For this review, use the dimensioned drawing (mm, ordinates from the lowest corner) and the shaded views. Coordinates: 2 decimals unless noted, no trailing zeros. Loops run counter-clockwise (first coordinate to the right, second up) from the corner with the lowest first, then second, coordinate; pieces in that order, holes last. Notation, with made-up numbers: M 11.25,22 L 35.25,22 A7 ccw 35.25,32 Z; hole C 72,-2.5 d10. An arc over 180 degrees is marked long. One line per item, written item: value.
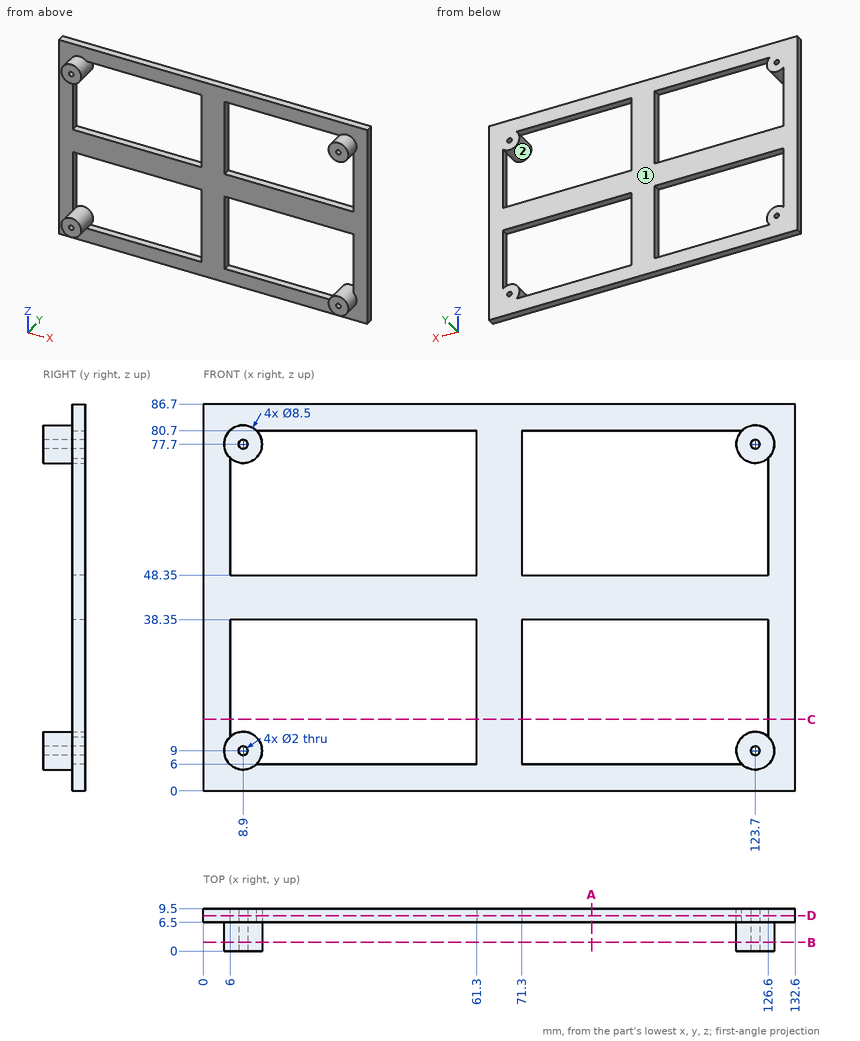
(1) Add section B-B on y = 2. State the section outline as (x, z) points.
Checks:
outline: C 8.9,9 d8.5; C 8.9,77.7 d8.5; C 123.7,9 d8.5; C 123.7,77.7 d8.5; hole C 8.9,9 d2; hole C 8.9,77.7 d2; hole C 123.7,9 d2; hole C 123.7,77.7 d2
(2) Add section A-A on x = 87. State the section outline as (y, z) points, then the cut area to 3 significant figures.
Checks:
outline: M 6.5,0 L 9.5,0 L 9.5,6 L 6.5,6 Z; M 6.5,38.35 L 9.5,38.35 L 9.5,48.35 L 6.5,48.35 Z; M 6.5,80.7 L 9.5,80.7 L 9.5,86.7 L 6.5,86.7 Z
area: 66.0 mm^2
(3) Draft analysis for pull direction Z (two halves, no side actions). For the marked faces 1 and 2, state which applies: pulls with the +Z half, pulls with the -Z half, needs draft (parallel to the pull), parting line crosses it, or undercut.
Checks:
face 1: needs draft
face 2: undercut
(4) To check wall thickness, follow L1, parallel to X at y = 7.5, z = 77.7; L2, parallel to Z at x = 8.9, y = 4.5; L3, parallel to Z at x = 92.5, y = 8. State the ranges of each line that lie inside material, in increasing order. Write a range as [from, to].
Checks:
L1: [0, 7.9], [9.9, 13.15], [61.3, 71.3], [119.45, 122.7], [124.7, 132.6]
L2: [4.75, 8], [10, 13.25], [73.45, 76.7], [78.7, 81.95]
L3: [0, 6], [38.35, 48.35], [80.7, 86.7]
(5) Add section D-D on y = 8. State how many separate pieces and enclosed holes the cut face has, then the cut area to 3 significant figures.
Checks:
separate pieces: 1
enclosed holes: 8
area: 4,510 mm^2
(6) Add section C-C on z = 16. State the section outline as (x, y) points.
Checks:
outline: M 0,6.5 L 6,6.5 L 6,9.5 L 0,9.5 Z; M 61.3,6.5 L 71.3,6.5 L 71.3,9.5 L 61.3,9.5 Z; M 126.6,6.5 L 132.6,6.5 L 132.6,9.5 L 126.6,9.5 Z
(7) Insertion check: pin 1 Ø1.2 at (x, z) = (123.7, 9) entering from +Y; pin 2 Ø3.5 at (y, z) = (8.5, 67.5) entering from -X; pin 3 Ø8 at (x, z) = (70.5, 43) entering from -Y. Each pin has a flat end and moves straight along its axis. Give the tip position at first contact, or say it passes through.
Checks:
pin 1: through
pin 2: x = 0
pin 3: y = 6.5
